Part print with two shaded views. Sizes in mm from the minimum x, y, z corner. A direction names the side the tool comes from. Give positions to 0.01 mm unless a question says otherwise; leave off trailing zeros. Order: outer loops, then holes, each group sorted by start corner. A loop starts at its lowest first (then second) coordinate and runs counter-clockwise, first axis right, second up.
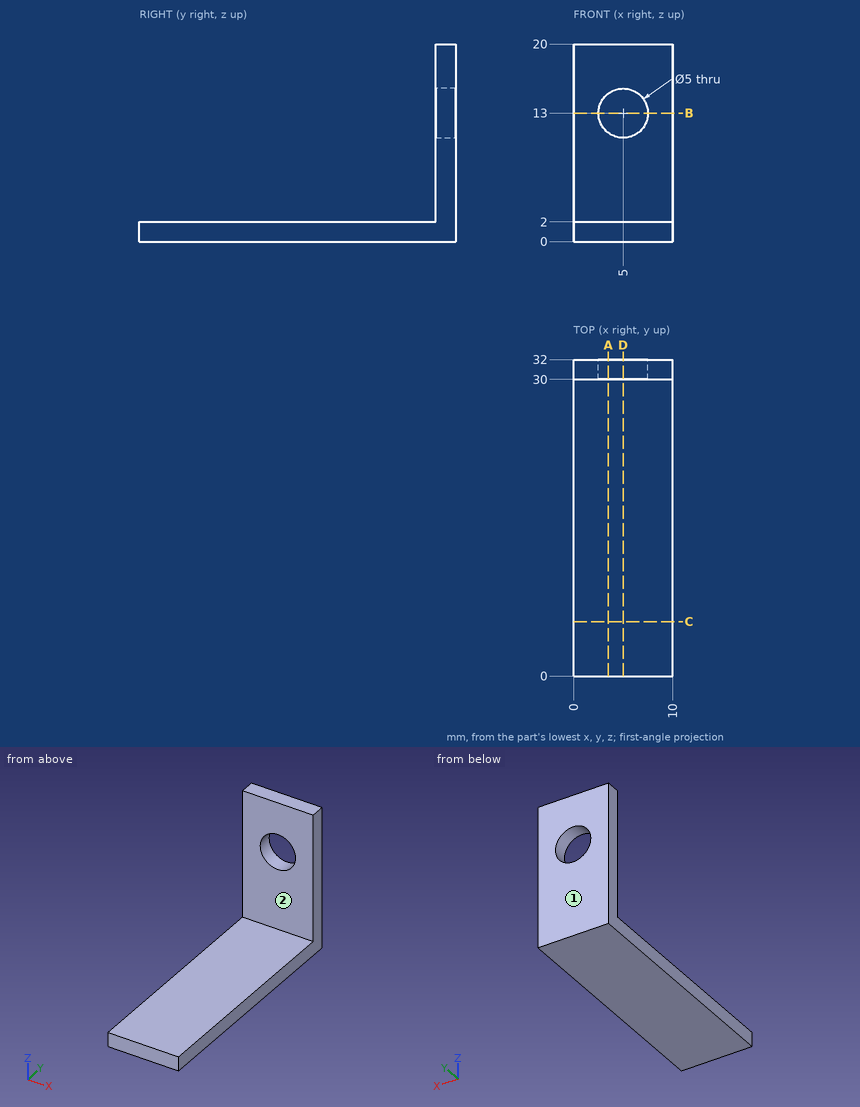
Item 1: Slice it at D-D (x = 5). Give the cut face in (y, z), and give its area (3 significant figures).
Item 2: Drop a flat-ended pin along its axis: pin 1 Ø3 at (x, z) = (5, 11.5) entering from -Y. Give the stop position or say it passes through.
Item 3: Wall check: L1, parallel to X at y = 30.7, z = 13; L2, parallel to Y at x = 7.5, z = 6.5; L3, parallel to Z at x = 9, y = 15.5. Give the ranges that are in metal, low to high.
Item 4: Slice it at A-A (x = 3.5). Give the cut face in (y, z).
Item 5: Slice it at B-B (z = 13). Give the cut face in (x, y), and give its area (3 significant figures).
Item 6: Tool access for the marked faces 1 and 2: list every direction of +Z, -Z, +X, -X, +Y, -Y with a clear straight run to the whole face (end or side of a thin tool).
Item 7: Slice it at C-C (y = 5.5). Give the cut face in (x, z), and give its area (3 significant figures).
A:
1. outline: (0, 0) - (32, 0) - (32, 10.5) - (30, 10.5) - (30, 2) - (0, 2) - close; (30, 15.5) - (32, 15.5) - (32, 20) - (30, 20) - close
1. area: 90.0 mm2
2. pin 1: stops at y = 30
3. L1: x = 0 to 2.5, 7.5 to 10
3. L2: y = 30 to 32
3. L3: z = 0 to 2
4. outline: (0, 0) - (32, 0) - (32, 11) - (30, 11) - (30, 2) - (0, 2) - close; (30, 15) - (32, 15) - (32, 20) - (30, 20) - close
5. outline: (0, 30) - (2.5, 30) - (2.5, 32) - (0, 32) - close; (7.5, 30) - (10, 30) - (10, 32) - (7.5, 32) - close
5. area: 10.0 mm2
6. face 1: +Z, -Z, +X, -X, +Y
6. face 2: +Z, +X, -X, -Y
7. outline: (0, 0) - (10, 0) - (10, 2) - (0, 2) - close
7. area: 20.0 mm2
